```python
from build123d import *

# Parameters (mm, degrees)
BOSS_EXTRUDE1_DEPTH      = 0.05
SKETCH2_W                = 200
SKETCH2_H                = 145
SKETCH2_W_2              = 15
BOSS_EXTRUDE2_DEPTH      = 0.1
BOSS_EXTRUDE3_DEPTH      = 0.05
SKETCH3_W                = 230
SKETCH3_H                = 1
BOSS_EXTRUDE7_DEPTH      = 0.03
BOSS_EXTRUDE7_DEPTH_BACK = 0.08
FILLET1_R                = 5
FILLET2_R                = 2


with BuildPart() as part:
    # Sketch1 → Boss-Extrude1 (new body)
    with BuildSketch(Plane(origin=(0, 0, 0), x_dir=(1, 0, 0), z_dir=(0, 1, 0))):
        with BuildLine():
            Line((-115, 80), (-115, -80))
            Line((-115, -80), (115, -80))
            Line((115, -80), (115, 80))
            Line((115, 80), (115, 105))
            ThreePointArc((115, 105), (113.535533906, 108.535533906), (110, 110))
            Line((110, 110), (-110, 110))
            ThreePointArc((-110, 110), (-113.535533906, 108.535533906), (-115, 105))
            Line((-115, 105), (-115, 80))
        make_face()
    extrude(amount=BOSS_EXTRUDE1_DEPTH)

    # Sketch2 → Boss-Extrude2 (add)
    with BuildSketch(Plane(origin=(0, 0.05, 0), x_dir=(1, 0, 0), z_dir=(0, 1, 0))):
        with Locations((0, -7.5)):
            Rectangle(SKETCH2_W, SKETCH2_H)
        with Locations((-107.5, -7.5)):
            Rectangle(SKETCH2_W_2, SKETCH2_H)
        with Locations((107.5, -7.5)):
            Rectangle(SKETCH2_W_2, SKETCH2_H)
    extrude(amount=BOSS_EXTRUDE2_DEPTH)

    # Sketch2_3 → Boss-Extrude3 (add)
    with BuildSketch(Plane(origin=(0, 0.05, 0), x_dir=(1, 0, 0), z_dir=(0, 1, 0))):
        Polygon((-115, 80), (-115, 65), (-100, 65), (-100, 71.339745962), align=None)
        Polygon((100, 71.339745962), (100, 65), (115, 65), (115, 80), align=None)
    extrude(amount=BOSS_EXTRUDE3_DEPTH)

    # Sketch3 → Boss-Extrude7 (add, two sides)
    with BuildSketch(Plane(origin=(0, 0.05, 0), x_dir=(1, 0, 0), z_dir=(0, 1, 0))) as boss_extrude7_sk:
        with Locations((0, 80)):
            Rectangle(SKETCH3_W, SKETCH3_H)
    extrude(amount=BOSS_EXTRUDE7_DEPTH)
    extrude(boss_extrude7_sk.sketch, amount=-BOSS_EXTRUDE7_DEPTH_BACK)

    # Fillet1
    fillet1_edges = [part.edges().sort_by_distance(p)[0] for p in [
        (115, 0.125, -65),
        (-115, 0.125, -65),
    ]]
    fillet(fillet1_edges, radius=FILLET1_R)

    # Fillet2
    fillet2_edges = [part.edges().sort_by_distance(p)[0] for p in [
        (-100, 0.075, -71.339745962),
        (100, 0.075, -71.339745962),
    ]]
    fillet(fillet2_edges, radius=FILLET2_R)


solid = part.part
```
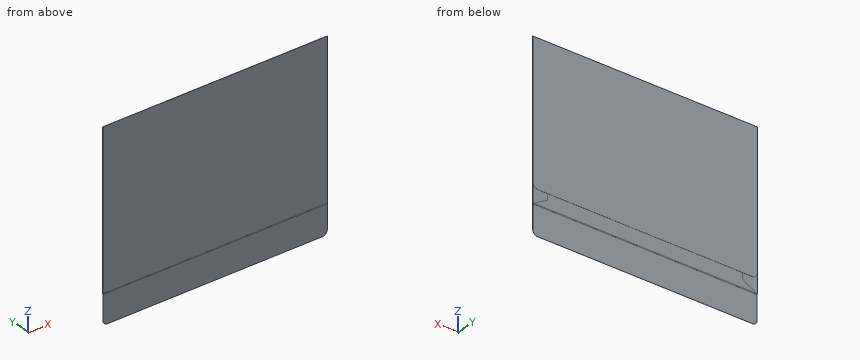
CAD build for the part. Positions are in the model's coordinates, mm. Round coordinates to 2 decimals unless told otherwise and drop trailing zeros. Write each loop counter-clockwise with the first axis right and the second up, starting at its lowest first coordinate (ties: lowest second). Pieces come first, ordered by that corner, then holes.
Item 1: Band-saw the part on C-C on z = -55. Write the cut outline in (x, y).
Filled in:
outline: (-115, 0) - (115, 0) - (115, 0.15) - (-115, 0.15) - close
Item 2: Band-saw the part on B-B on z = -93.5. Write the cut outline in (x, y).
Filled in:
outline: (-115, 0) - (115, 0) - (115, 0.05) - (-115, 0.05) - close
Item 3: Drop flat-ended pins along their axis: pin 1 Ø10 at (x, z) = (-66.5, 26.5) entering from -Y; pin 2 Ø9 at (x, z) = (1, -96.5) entering from +Y. Give the stop position or say it passes through.
Filled in:
pin 1: stops at y = 0
pin 2: stops at y = 0.05
Item 4: Drill centre line: L1, parallel to Y at x = -54.5, z = -23.5. Where is it in solid material? Low to high.
Filled in:
L1: y = 0 to 0.15
